Verification items for the finished model (mm, model axes). Face numbers are marked on the shaded views. A direction names the side the tool comes from. Round coordinates to 2 decimals unless told otherwise and drop trailing zeros. Order: outer loops, then holes, each group sorted by start corner. A loop starts at its lowest first (then second) coordinate and runs counter-clockwise, first axis right, second up. Notation, with made-up numbers: (52.5, 17.5) -> (104.5, 17.5) arc R7 ccw to (104.5, 23.5) -> close; hole circle Ø4 at (59.25, 21.5). An arc over 180 degrees is marked (long way). Answer in a Markdown table with one row per item. Add a question column.
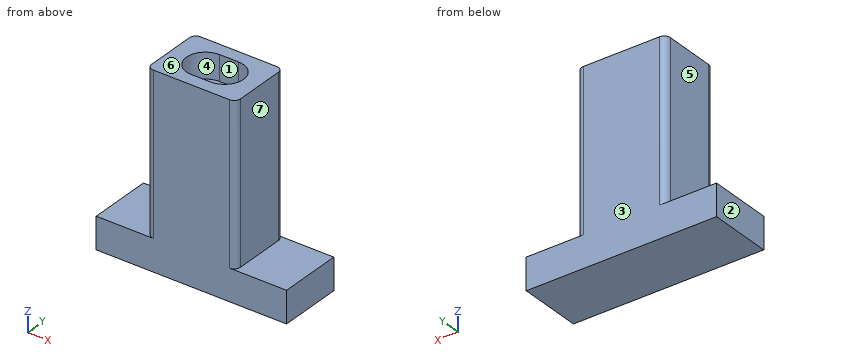
```python
from build123d import *

# Parameters (mm, degrees)
SKETCH_W           = 30
SKETCH_H           = 10
PAD_DEPTH          = 30
POCKET_DEPTH       = 4
SKETCH003_W        = 15
SKETCH003_H        = 10
POCKET001_DEPTH    = 25
POLARPATTERN_COUNT = 2
FILLET_R           = 1


with BuildPart() as part:
    # Sketch → Pad (new body)
    with BuildSketch(Plane.XY):
        Rectangle(SKETCH_W, SKETCH_H)
    extrude(amount=PAD_DEPTH)

    # Sketch001 → Pocket (cut)
    with BuildSketch(Plane.XY.offset(30)):
        with BuildLine():
            ThreePointArc((-1.5, 3), (-4.5, 0), (-1.5, -3))
            Line((-1.5, -3), (1.5, -3))
            ThreePointArc((1.5, -3), (4.5, 0), (1.5, 3))
            Line((-1.5, 3), (1.5, 3))
        make_face()
    extrude(amount=-POCKET_DEPTH, mode=Mode.SUBTRACT)

    # Sketch003 → Pocket001 (cut)
    with BuildSketch(Plane.XY.offset(30)):
        with Locations((14.5, 0)):
            Rectangle(SKETCH003_W, SKETCH003_H)
    pocket001 = extrude(amount=-POCKET001_DEPTH, mode=Mode.SUBTRACT)

    # PolarPattern: Pocket001 ×2 about axis
    polarpattern_axis = Axis((0, 0, 30), (0, 0, 1))
    for i in range(1, POLARPATTERN_COUNT):
        add(pocket001.rotate(polarpattern_axis, i * 360 / POLARPATTERN_COUNT), mode=Mode.SUBTRACT)

    # Fillet
    fillet_edges = [part.edges().sort_by_distance(p)[0] for p in [
        (-7, 5, 17.5),
        (-7, -5, 17.5),
        (7, -5, 17.5),
        (7, 5, 17.5),
    ]]
    fillet(fillet_edges, radius=FILLET_R)


solid = part.part
```
1) Cross-section at D-D, the plane x = -2. Record the boundary of the cut face in (y, z), and give its area (3 significant figures).
2) Cross-section at B-B, the plane y = 0. Record the boundary of the cut face in (x, z).
3) Cross-section at C-C, the plane z = 21. Record the boundary of the cut face in (x, y), and give its area (3 significant figures).
4) Depth check by flat-ended pin: P1, Ø3, axis at y = -3, z = 15.5, coming from the -X side; P2, Ø10, axis at x = -9, z = 22.5, coming from the -Y side; P3, Ø4.5, axis at x = -12, y = 0.5, coming from the +Z side; P4, Ø6, axis at y = 1, z = 18, coming from the +X side. Enter the tip coordinate at first touch or a pass-through.
5) Tool access check on the marked faces 5, 6 and 7. Record the directions out of +Z, -Z, +X, -X, +Y, -Y that give a thin tool (end or side, any length) a straight path to the whole face; none if there is none.
6) Thickness scan on L1, parallel to X at y = -0.25, z = 21; L2, parallel to Y at x = 3, z = 28; L3, parallel to Z at x = -9.75, y = 0.5. Record the ranges inside material, lowest first. Write a range as [from, to].
7) Cross-section at A-A, the plane z = 27.75. Record the boundary of the cut face in (x, y).
8) Draft check along Y on the marked faces 1, 2, 3 and 4. Enter one of: +Y half, -Y half, draft (parallel to the pull), parting line (faces both ways), or undercut.
Results below:
| question | item | result |
|---|---|---|
| 1 | outline | (-5, 0) -> (5, 0) -> (5, 30) -> (2.96, 30) -> (2.96, 26) -> (-2.96, 26) -> (-2.96, 30) -> (-5, 30) -> close |
| 1 | area | 276 mm² |
| 2 | outline | (-15, 0) -> (15, 0) -> (15, 5) -> (7, 5) -> (7, 30) -> (4.5, 30) -> (4.5, 26) -> (-4.5, 26) -> (-4.5, 30) -> (-7, 30) -> (-7, 5) -> (-15, 5) -> close |
| 3 | outline | (-7, -4) arc R1 ccw to (-6, -5) -> (6, -5) arc R1 ccw to (7, -4) -> (7, 4) arc R1 ccw to (6, 5) -> (-6, 5) arc R1 ccw to (-7, 4) -> close |
| 3 | area | 139 mm² |
| 4 | P1 | x = -7 |
| 4 | P2 | y = -5 |
| 4 | P3 | z = 5 |
| 4 | P4 | x = 7 |
| 5 | face 5 | +Z, -X, +Y, -Y |
| 5 | face 6 | +Z, +X, -X, +Y, -Y |
| 5 | face 7 | +Z, +X, +Y, -Y |
| 6 | L1 | [-7, 7] |
| 6 | L2 | [-5, -2.6], [2.6, 5] |
| 6 | L3 | [0, 5] |
| 7 | outline | (-7, -4) arc R1 ccw to (-6, -5) -> (6, -5) arc R1 ccw to (7, -4) -> (7, 4) arc R1 ccw to (6, 5) -> (-6, 5) arc R1 ccw to (-7, 4) -> close; hole (-1.5, -3) -> (1.5, -3) arc R3 ccw to (1.5, 3) -> (-1.5, 3) arc R3 ccw to start |
| 8 | face 1 | undercut |
| 8 | face 2 | draft |
| 8 | face 3 | +Y half |
| 8 | face 4 | undercut |
